from build123d import *

# Parameters (mm, degrees)
ESQUISSE1_W             = 440
ESQUISSE1_H             = 150
BOSS_EXTRU_1_DEPTH      = 4
ESQUISSE2_W             = 4
ESQUISSE2_H             = 60
ENL_V_MAT_EXTRU_1_DEPTH = 4
ESQUISSE3_W             = 50
ESQUISSE3_H             = 4
BOSS_EXTRU_2_DEPTH      = 4
ENL_V_MAT_EXTRU_2_DEPTH = 10
ESQUISSE5_R             = 1.6
ENL_V_MAT_EXTRU_3_DEPTH = 4


with BuildPart() as part:
    # Esquisse1 → Boss.-Extru.1 (new body)
    with BuildSketch(Plane.XY):
        Rectangle(ESQUISSE1_W, ESQUISSE1_H)
    extrude(amount=BOSS_EXTRU_1_DEPTH)

    # Esquisse2 → Enlèv. mat.-Extru.1 (cut)
    with BuildSketch(Plane.XY.offset(4)):
        with Locations((-218, 0)):
            Rectangle(ESQUISSE2_W, ESQUISSE2_H)
        with Locations((218, 0)):
            Rectangle(ESQUISSE2_W, ESQUISSE2_H)
    extrude(amount=-ENL_V_MAT_EXTRU_1_DEPTH, mode=Mode.SUBTRACT)

    # Esquisse3 → Boss.-Extru.2 (add)
    with BuildSketch(Plane.XY.offset(4)):
        with Locations((-95, -77)):
            Rectangle(ESQUISSE3_W, ESQUISSE3_H)
        with Locations((95, -77)):
            Rectangle(ESQUISSE3_W, ESQUISSE3_H)
        with Locations((95, 77)):
            Rectangle(ESQUISSE3_W, ESQUISSE3_H)
        with Locations((-95, 77)):
            Rectangle(ESQUISSE3_W, ESQUISSE3_H)
    extrude(amount=-BOSS_EXTRU_2_DEPTH)

    # Esquisse4 → Enlèv. mat.-Extru.2 (cut)
    with BuildSketch(Plane.XY.offset(4)):
        Polygon((132.4, 75), (135.6, 75), (135.6, 72), (136.85, 72), (136.85, 67.8), (135.6, 67.8), (135.6, 64), (132.4, 64), (132.4, 67.8), (131.15, 67.8), (131.15, 72), (132.4, 72), align=None)
        Polygon((54.4, 75), (57.6, 75), (57.6, 72), (58.85, 72), (58.85, 67.8), (57.6, 67.8), (57.6, 64), (54.4, 64), (54.4, 67.8), (53.15, 67.8), (53.15, 72), (54.4, 72), align=None)
        Polygon((-56.849728223, 75), (-53.649728223, 75), (-53.649728223, 72), (-52.399728223, 72), (-52.399728223, 67.8), (-53.649728223, 67.8), (-53.649728223, 64), (-56.849728223, 64), (-56.849728223, 67.8), (-58.099728223, 67.8), (-58.099728223, 72), (-56.849728223, 72), align=None)
        Polygon((-134.849728223, 75), (-131.649728223, 75), (-131.649728223, 72), (-130.399728223, 72), (-130.399728223, 67.8), (-131.649728223, 67.8), (-131.649728223, 64), (-134.849728223, 64), (-134.849728223, 67.8), (-136.099728223, 67.8), (-136.099728223, 72), (-134.849728223, 72), align=None)
        Polygon((-131.649728223, -75), (-131.649728223, -72), (-130.399728223, -72), (-130.399728223, -67.8), (-131.649728223, -67.8), (-131.649728223, -64), (-134.849728223, -64), (-134.849728223, -67.8), (-136.099728223, -67.8), (-136.099728223, -72), (-134.849728223, -72), (-134.849728223, -75), align=None)
        Polygon((-53.649728223, -75), (-53.649728223, -72), (-52.399728223, -72), (-52.399728223, -67.8), (-53.649728223, -67.8), (-53.649728223, -64), (-56.849728223, -64), (-56.849728223, -67.8), (-58.099728223, -67.8), (-58.099728223, -72), (-56.849728223, -72), (-56.849728223, -75), align=None)
        Polygon((57.6, -75), (57.6, -72), (58.85, -72), (58.85, -67.8), (57.6, -67.8), (57.6, -64), (54.4, -64), (54.4, -67.8), (53.15, -67.8), (53.15, -72), (54.4, -72), (54.4, -75), align=None)
        Polygon((135.6, -75), (135.6, -72), (136.85, -72), (136.85, -67.8), (135.6, -67.8), (135.6, -64), (132.4, -64), (132.4, -67.8), (131.15, -67.8), (131.15, -72), (132.4, -72), (132.4, -75), align=None)
    extrude(amount=-ENL_V_MAT_EXTRU_2_DEPTH, mode=Mode.SUBTRACT)

    # Esquisse5 → Enlèv. mat.-Extru.3 (cut)
    with BuildSketch(Plane.XY.offset(4)):
        with Locations((218, -50)):
            Circle(ESQUISSE5_R)
        with Locations((218, 50)):
            Circle(ESQUISSE5_R)
        with Locations(Location((-218, 50, 0), (0, 0, 180))):
            Circle(ESQUISSE5_R)
        with Locations(Location((-218, -50, 0), (0, 0, 180))):
            Circle(ESQUISSE5_R)
    extrude(amount=-ENL_V_MAT_EXTRU_3_DEPTH, mode=Mode.SUBTRACT)


solid = part.part
Design review of the part built by this model. Coordinates are the model's own, in mm. Round coordinates to 2 decimals unless told otherwise and drop trailing zeros. Order: outer loops, then holes, each group sorted by start corner. A loop starts at its lowest first (then second) coordinate and runs counter-clockwise, first axis right, second up.
1) Consider section A-A (z = 1.1). Count the separate pieces of the cut face and the enclosed holes in it, plus the area to 3 significant figures.
The answers:
separate pieces: 1
enclosed holes: 4
area: 65,900 mm2
2) For L1, parallel to Y at x = 218, z = 1.1; L2, parallel to X at y = -71.5, z = 1.9; L3, parallel to X at y = -50.5, z = 2.6, list the stretches that pass through material, from the lowest coordinate up.
The answers:
L1: y = -75 to -51.6, -48.4 to -30, 30 to 48.4, 51.6 to 75
L2: x = -220 to -136.1, -130.4 to -58.1, -52.4 to 53.15, 58.85 to 131.15, 136.85 to 220
L3: x = -220 to -219.52, -216.48 to 216.48, 219.52 to 220
3) Consider section C-C (x = 14). State the section outline as (y, z) points, plus the area to 3 significant figures.
The answers:
outline: (-75, 0) - (75, 0) - (75, 4) - (-75, 4) - close
area: 600 mm2
4) Clearance check with flat-ended pins moving along their axes: pin 1 Ø0.6 at (x, z) = (-131, 2) entering from +Y; pin 2 Ø1 at (x, z) = (-53, 2.5) entering from -Y; pin 3 Ø1.6 at (x, z) = (134, 2) entering from +Y. State where each tip first meets the part, or that it passes through.
The answers:
pin 1: stops at y = 75
pin 2: stops at y = -75
pin 3: stops at y = 64
5) Consider section B-B (y = -10.5). State the section outline as (x, z) points.
The answers:
outline: (-216, 0) - (216, 0) - (216, 4) - (-216, 4) - close
